```python
from build123d import *

# Parameters (mm, degrees)
F3_R        = 25
F4_DEPTH    = 1
F5_W        = 1.1802830268
F5_H        = 5.150327459
F6_DEPTH    = 5
F7_R        = 4.99999
F8_T1_DEPTH = 9.8176261194


# Not quite as in the source:
# - a fillet or chamfer that OpenCascade refuses, or shapes differently, is made with other operations: its cross-section is extruded or revolved along the edge and cut away or added
# - a fillet or chamfer is up to 0.001 mm smaller than in the source, because OpenCascade refuses the exact size


with BuildPart() as f1:
    # F0 (on Front) → F1 (revolve)
    with BuildSketch(Plane.XZ):
        with BuildLine():
            Line((-30, 0), (0, 0))
            Line((0, 0), (0, 3))
            Line((0, 3), (-25, 3))
            ThreePointArc((-25, 3), (-27.9154759474, 2.1924599124), (-30, 0))
        make_face()
    revolve(axis=Axis((0, 0, 1.5), (0, 0, 1)))

    # F3 (on face) → F4 (join)
    with BuildSketch(Plane.XY.offset(3)):
        Circle(F3_R)
    extrude(amount=F4_DEPTH)

    # F5 (on face) → F6 (join)
    with BuildSketch(Plane.XY.offset(4)):
        with Locations((-3.5133393249, 19.3324619904)):
            Rectangle(F5_W, F5_H)
    extrude(amount=F6_DEPTH)

    # F7 (radius 5 in the source; OpenCascade refuses exactly that, so slightly less here)
    f7_edges = [f1.edges().sort_by_distance(p)[0] for p in [
        (-3.513339, 21.907626, 9),
    ]]
    fillet(f7_edges, radius=F7_R)

    # F8: fillet of radius 10 on 1 edges, made by hand

    # F8_s2 → F8_t1 (cut)
    with BuildSketch(Plane.YZ.offset(-8.4221523845)):
        with BuildLine():
            ThreePointArc((16.9076357199, 9), (16.7949535216, 8.1395303981), (16.7572982609, 7.2725313815))
            Line((16.7572982609, 7.2725313815), (16.7572982609, 9))
            Line((16.7572982609, 9), (16.9076357199, 9))
        make_face()
    extrude(amount=F8_T1_DEPTH, mode=Mode.SUBTRACT)


solid = f1.part
```
Check sheet for the modelled part. Datum: model origin and axes. Units: mm. A direction names the side the tool comes from. Round coordinates to 2 decimals unless told otherwise and drop trailing zeros. Loops run counter-clockwise (first coordinate to the right, second up) from the corner with the lowest first, then second, coordinate; pieces in that order, holes last. Notation, with made-up numbers: (-36.75, -24.75) -> (-16.75, -24.75) arc R15 ccw to (-16.75, 0.25) -> close; hole circle Ø5 at (-23.5, 3). An arc over 180 degrees is marked (long way). Write item = value, one per line. Start each with the question number.
1) Sectioned sample at C-C, the plane z = 8. Record the cut outline in (x, y), plus the area to 3 significant figures.
2) Set-up check for faces 1 (the cylindrical face through (-3.51, 20.48, 7.5)), 2 (the flat face through (-2.923, 19, 6)), 3 (the flat face through (0, 0, 0)), 4 (the flat face through (-4.103, 19, 6)), 5 (the cylindrical face through (23.846, 7.509, 3.493)): record each of +Z, -Z, +X, -X, +Y, -Y from which the full face is reachable in a straight line by a thin tool's end or side.
3) Sectioned sample at D-D, the plane z = 1.5. Record the cut outline in (x, y).
4) Gauge pin test, flat ends, axial feed: pin 1 Ø1.5 at (y, z) = (2.5, 3) entering from +X; pin 2 Ø3 at (x, y) = (-24, -1) entering from +Z; pin 3 Ø4 at (y, z) = (18, 6.5) entering from +X. Record the tip position at first contact, or that the pin passes through.
5) Thickness scan on probe 1 along Z at (x, y) = (3, -17); probe 2 along Y at (x, z) = (-15, 2.25); probe 3 along Y at (x, z) = (-27, 0.5). Record the ranges inside material, lowest first.
6) Sectioned sample at A-A, the plane y = 0. Record the cut outline in (x, z).
Results are:
q1.outline = (-4.1, 16.78) -> (-2.92, 16.78) -> (-2.92, 19.91) -> (-4.1, 19.91) -> close
q1.area = 3.69 mm^2
q2.face_1 = +Z, +X, -X, +Y
q2.face_2 = +Z, +X, +Y, -Y
q2.face_3 = -Z, +X, -X, +Y, -Y
q2.face_4 = +Z, -X, +Y, -Y
q2.face_5 = +Z
q3.outline = circle Ø57.68 at (0, 0)
q4.pin_1 = 27.71
q4.pin_2 = 4
q4.pin_3 = -2.92
q5.probe_1 = 0 to 4
q5.probe_2 = -23.43 to 23.43
q5.probe_3 = -12.37 to 12.37
q6.outline = (-30, 0) -> (30, 0) arc R5.67 ccw to (25, 3) -> (25, 4) -> (-25, 4) -> (-25, 3) arc R5.67 ccw to start
